```python
from build123d import *

# Parameters (mm, degrees)
F1_DEPTH = 40
F2_T     = -3


with BuildPart() as f1:
    # F0 (on Front) → F1 (new body)
    with BuildSketch(Plane.XZ):
        with BuildLine():
            Line((0, 0.086318), (0, -119.913682))
            ThreePointArc((0, -119.913682), (84.852814, -84.766496), (120, 0.086318))
            Line((120, 0.086318), (0, 0.086318))
        make_face()
    extrude(amount=F1_DEPTH)

    # F2
    f2_openings = [f1.faces().sort_by_distance(p)[0] for p in [
        (50.929582, -40, -50.843264),
    ]]
    offset(amount=F2_T, openings=f2_openings)


solid = f1.part
```
Input: part model. Units: mm. Frame: model coordinates. A direction names the side the tool comes from. Give positions to 0.01 mm unless a question says otherwise; leave off trailing zeros. Write each loop counter-clockwise with the first axis right and the second up, starting at its lowest first coordinate (ties: lowest second). Pieces come first, ordered by that corner, then holes. Notation, with made-up numbers: (22.5, 52.5) - (57.5, 52.5) arc R24 cw to (57.5, 69.5) - close; hole circle Ø1 at (-26.75, -30). An arc over 180 degrees is marked (long way). Write item = value, one per line. Start each with the question number.
1) Cut plane B-B (z = -8). Return loops of the section in (x, y).
2) Cut plane C-C (x = 19.5). Return loops of the section in (y, z), and give its area (3 significant figures).
3) Reachability of faces 1 (the face through (61, -21, -2.914)), 2 (the face through (0, -20, -59)) from +Z, -Z, +X, -X, +Y, -Y: full face, straight path, thin tool, end or side. Return the list, or none.
4) Cut plane A-A (y = -12.5). Return loops of the section in (x, z).
5) Pin query (flat end, axial travel): pin 1 (4 mm diameter, centred on y = -9, z = -29, fed in from +X); pin 2 (18.5 mm diameter, centred on y = -13, z = -84, fed in from +X); pin 3 (10 mm diameter, centred on x = 49, z = -49, fed in from -Y). Return the tip coordinate at first contact, or that it passes through.
6) Material intervals for L1, parallel to Y at x = 8, z = -26; L2, parallel to Z at x = 29.5, y = -6.5; L3, parallel to Z at x = 28, y = -4.5, sorted ascending. Write a range as [from, to].
7) Draft query along Z for faces 3 (the face through (47, -3, -46)), 4 (the face through (61, -20, 0.086)), 5 (the face through (3, -21, -59)), 6 (the face through (2, -40, -46)). Return one class per face: pulls with the +Z half, pulls with the -Z half, needs draft (parallel to the pull), parting line crosses it, or undercut.
Answers follow:
q1.outline = (0, -40) - (3, -40) - (3, -3) - (116.72, -3) - (116.72, -40) - (119.73, -40) - (119.73, 0) - (0, 0) - close
q2.outline = (-40, -118.32) - (0, -118.32) - (0, 0.09) - (-40, 0.09) - (-40, -2.91) - (-3, -2.91) - (-3, -115.28) - (-40, -115.28) - close
q2.area = 579 mm^2
q3.face_1 = -Y
q3.face_2 = +Z, -Z, -X, +Y, -Y
q4.outline = (0, -119.91) arc R120 ccw to (120, 0.09) - (0, 0.09) - close; hole (3, -116.88) arc R117 ccw to (116.96, -2.91) - (3, -2.91) - close
q5.pin_1 = 116.9
q5.pin_2 = 93.81
q5.pin_3 = -3
q6.L1 = [-3, 0]
q6.L2 = [-116.23, -113.13], [-2.91, 0.09]
q6.L3 = [-116.6, -113.51], [-2.91, 0.09]
q7.face_3 = undercut
q7.face_4 = pulls with the +Z half
q7.face_5 = undercut
q7.face_6 = needs draft
